Can you work these out from the drawing? Everything is in mm from the part's minimum corner. A direction names the side the tool comes from. Give positions to 0.01 mm unless a question says otherwise; leave off trailing zeros. Loops run counter-clockwise (first coordinate to the right, second up) from the corner with the lowest first, then second, coordinate; pieces in that order, holes last. Notation, with made-up numbers: M 36.25,73.5 L 71.25,73.5 A24 cw 71.25,111.5 Z; hole C -6,61.25 d2. An arc over 180 degrees is marked long. Use CSV: the item, a comma, the result in double quotes.
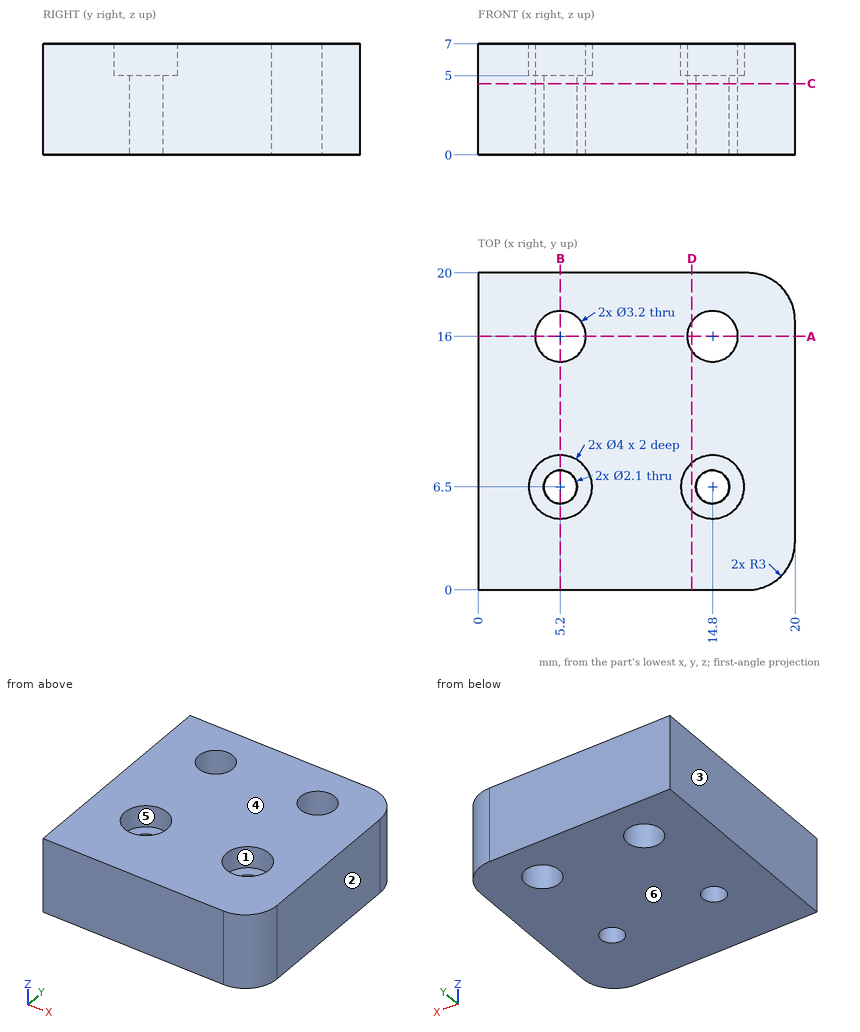
Q1. Please list where these lines run through material, in increasing order: L1, parallel to Y at x = 14.8, z = 2.2; L2, parallel to X at y = 15, z = 5.25; L3, parallel to Y at x = 3.75, z = 6. Write a range as from..to.
Model answer:
L1,"0..5.45, 7.55..14.4, 17.6..20"
L2,"0..3.95, 6.45..13.55, 16.05..20"
L3,"0..5.12, 7.88..15.32, 16.68..20"
Q2. For the marked faces 5 and 6, which set-ups out of +Z, -Z, +X, -X, +Y, -Y let a thin tool reach every point of the face, with its end or its side?
Model answer:
face 5,"+Z"
face 6,"-Z, +X, -X, +Y, -Y"
Q3. I want a section at C-C, the plane z = 4.5. Please give me the cut outline in (x, y).
Model answer:
outline,"M 0,0 L 17,0 A3 ccw 20,3 L 20,17 A3 ccw 17,20 L 0,20 Z; hole C 5.2,16 d3.2; hole C 5.2,6.5 d2.1; hole C 14.8,16 d3.2; hole C 14.8,6.5 d2.1"
Q4. If we mould it in two halves opening along X, with no side actions, what happens to the marked faces 1, 2, 3 and 4? For each: released by +X, released by -X, zero draft, split by the parting line, or undercut.
Model answer:
face 1,"undercut"
face 2,"released by +X"
face 3,"released by -X"
face 4,"zero draft"
Q5. I want a section at B-B, the plane x = 5.2. Please give me the cut outline in (y, z).
Model answer:
outline,"M 0,0 L 5.45,0 L 5.45,5 L 4.5,5 L 4.5,7 L 0,7 Z; M 7.55,0 L 14.4,0 L 14.4,7 L 8.5,7 L 8.5,5 L 7.55,5 Z; M 17.6,0 L 20,0 L 20,7 L 17.6,7 Z"
Q6. I want a section at A-A, the plane y = 16. Please give me the cut outline in (x, z).
Model answer:
outline,"M 0,0 L 3.6,0 L 3.6,7 L 0,7 Z; M 6.8,0 L 13.2,0 L 13.2,7 L 6.8,7 Z; M 16.4,0 L 20,0 L 20,7 L 16.4,7 Z"
Q7. I'm going to push a flat-ended pin straight in: P1, Ø2.5, axis at x = 5.2, y = 6.5, coming from the +Z side. Where does the tip first touch, or does it pass through?
Model answer:
P1,"z = 5"
Q8. I want a section at D-D, the plane x = 13.5. Please give me the cut outline in (y, z), then the cut area to 3 significant figures.
Model answer:
outline,"M 0,0 L 15.07,0 L 15.07,7 L 8.02,7 L 8.02,5 L 4.98,5 L 4.98,7 L 0,7 Z; M 16.93,0 L 20,0 L 20,7 L 16.93,7 Z"
area,"121 mm2"
